from build123d import *

# Parameters (mm, degrees)
F2_W     = 0.998062
F2_H     = 0.0508
F2_W_2   = 0.0508
F2_H_2   = 0.998062
F3_DEPTH = 8.636
F4_W     = 0.8
F4_H     = 0.0508
F4_W_2   = 0.0508
F4_H_2   = 0.8
F5_DEPTH = 1.9304


with BuildPart() as f1:
    # F0 (on Right) → F1 (revolve)
    with BuildSketch(Plane.YZ):
        with BuildLine():
            Line((2.4765, 8.636), (2.4765, 0))
            Line((2.4765, 0), (3.2639, 0))
            Line((3.2639, 0), (3.2639, 1.1938))
            Line((3.2639, 1.1938), (3.81, 1.1938))
            ThreePointArc((3.81, 1.1938), (4.708026, 1.565774), (5.08, 2.4638))
            Line((5.08, 2.4638), (5.08, 8.382))
            ThreePointArc((5.08, 8.382), (4.708026, 9.280026), (3.81, 9.652))
            Line((3.81, 9.652), (2.4511, 9.652))
            Line((2.4511, 9.652), (2.4511, 11.43))
            Line((2.4511, 11.43), (1.6002, 11.43))
            Line((1.6002, 11.43), (1.6002, 9.4996))
            Line((1.6002, 9.4996), (0, 9.4996))
            Line((0, 9.4996), (0, 8.636))
            Line((0, 8.636), (2.4765, 8.636))
        make_face()
    revolve(axis=Axis((0, 0, 4.318), (0, 0, -1)))

    # F2 (on face) → F3 (join, through all)
    with BuildSketch(Plane(origin=(0, 0, 0), x_dir=(1, 0, 0), z_dir=(0, 0, -1))):
        with Locations((0, 2.4511)):
            Rectangle(F2_W, F2_H)
        with Locations((2.4511, 0)):
            Rectangle(F2_W_2, F2_H_2)
        with Locations((0, -2.4511)):
            Rectangle(F2_W, F2_H)
        with Locations((-2.4511, 0)):
            Rectangle(F2_W_2, F2_H_2)
    extrude(amount=-F3_DEPTH)

    # F4 (on face) → F5 (join, through all)
    with BuildSketch(Plane.XY.offset(11.43)):
        with Locations((0, -1.5748)):
            Rectangle(F4_W, F4_H)
        with Locations((-1.5748, 0)):
            Rectangle(F4_W_2, F4_H_2)
        with Locations((0, 1.5748)):
            Rectangle(F4_W, F4_H)
        with Locations((1.5748, 0)):
            Rectangle(F4_W_2, F4_H_2)
    extrude(amount=-F5_DEPTH)


solid = f1.part
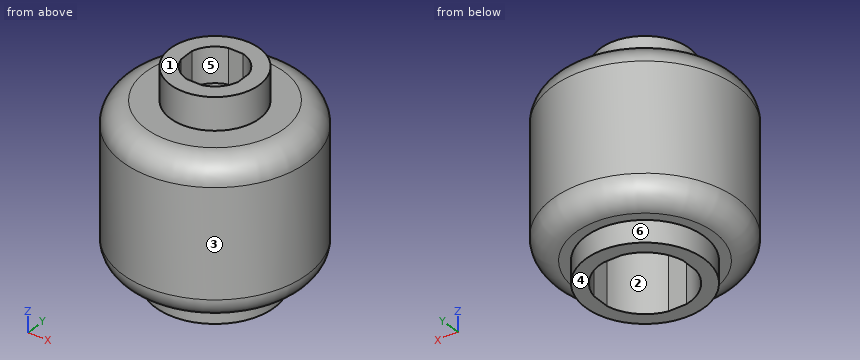
Verification items for the finished model (mm, model axes). Face numbers are marked on the shaded views. A direction names the side the tool comes from. Give positions to 0.01 mm unless a question says otherwise; leave off trailing zeros. Write each loop counter-clockwise with the first axis right and the second up, starting at its lowest first coordinate (ties: lowest second). Pieces come first, ordered by that corner, then holes.
(1) Mould release check, pull along Y, two halves, no side actions. Record for the marked faces 1, 2 and 3: +Y half, -Y half, draft (parallel to the pull), parting line (faces both ways), or undercut.
(2) Cross-section at A-A (z = 5.75). Enter the section's corners in (x, y), plus the area to 3 significant figures.
(3) Access from +Z, -Z, +X, -X, +Y, -Y to the whole of each face (thin tool, end or side, straight path). Record for the marked faces 4, 5 and 6.
(4) Cross-section at D-D (z = 10.75). Enter the section's corners in (x, y).
(5) Cross-section at B-B (y = 0). Enter the section's corners in (x, z), plus the area to 3 significant figures.
(6) Gauge pin test, flat ends, axial feed: pin 1 (4 mm diameter, centred on x = 2, z = 10, fed in from +Y); pin 2 (1.5 mm diameter, centred on x = 1, z = 6, fed in from +Y). Record the tip position at first contact, or that the pin passes through.
(7) Material ranges on line 1 (X direction, y = 0, z = 11); line 2 (Z direction, x = -0.5, y = 3.5); line 3 (X direction, y = -1.5, z = 2.75), recorded low to high.
Worked out:
1. face 1: draft
1. face 2: undercut
1. face 3: parting line
2. outline: circle Ø10.16 at (0, 0); hole (-2.43, -0.5) arc R2.48 ccw to (-0.5, -2.43) - (0.5, -2.43) arc R2.48 ccw to (2.43, -0.5) - (2.43, 0.5) arc R2.48 ccw to (0.5, 2.43) - (-0.5, 2.43) arc R2.48 ccw to (-2.43, 0.5) - close
2. area: 61.9 mm2
3. face 4: -Z, +X, -X, +Y, -Y
3. face 5: +Z
3. face 6: -Z
4. outline: circle Ø4.9 at (0, 0); hole (-1.55, -0.4) arc R1.6 ccw to (-0.4, -1.55) - (0.4, -1.55) arc R1.6 ccw to (1.55, -0.4) - (1.55, 0.4) arc R1.6 ccw to (0.4, 1.55) - (-0.4, 1.55) arc R1.6 ccw to (-1.55, 0.4) - close
5. outline: (-5.08, 2.46) arc R1.27 ccw to (-3.81, 1.19) - (-3.26, 1.19) - (-3.26, 0) - (-2.43, 0) - (-2.43, 8.64) - (2.43, 8.64) - (2.43, 0) - (3.26, 0) - (3.26, 1.19) - (3.81, 1.19) arc R1.27 ccw to (5.08, 2.46) - (5.08, 8.38) arc R1.27 ccw to (3.81, 9.65) - (2.45, 9.65) - (2.45, 11.43) - (1.55, 11.43) - (1.55, 9.5) - (-1.55, 9.5) - (-1.55, 11.43) - (-2.45, 11.43) - (-2.45, 9.65) - (-3.81, 9.65) arc R1.27 ccw to (-5.08, 8.38) - close
5. area: 53.2 mm2
6. pin 1: stops at y = 5.03
6. pin 2: stops at y = 5.07
7. line 1: x = -2.45 to -1.55, 1.55 to 2.45
7. line 2: z = 1.19 to 9.65
7. line 3: x = -4.85 to -1.97, 1.97 to 4.85
